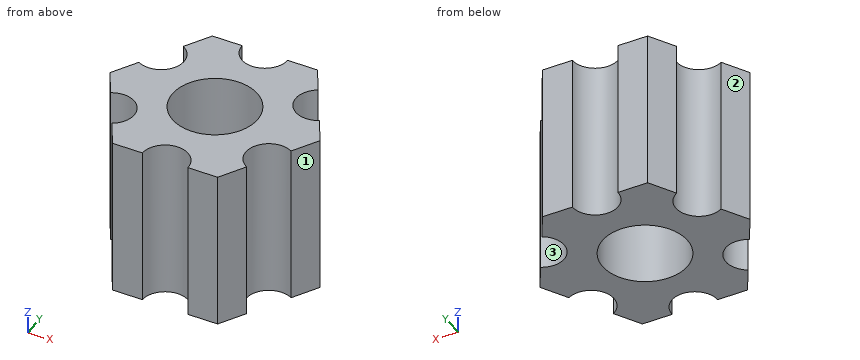
```python
from build123d import *

# Parameters (mm, degrees)
SKETCH1_R           = 2.9337
BOSS_EXTRUDE1_DEPTH = 15.875
CUT_EXTRUDE1_DEPTH  = 4.7625


with BuildPart() as part:
    # Sketch1 → Boss-Extrude1 (new body)
    with BuildSketch(Plane(origin=(0, 0, 0), x_dir=(-1, 0, 0), z_dir=(0, 0, -1))):
        with BuildLine():
            Line((-4.70551159, -4.549815043), (-3.666174521, -6.349999904))
            Line((-3.666174521, -6.349999904), (-1.587500385, -6.349999904))
            ThreePointArc((-1.587500385, -6.349999904), (-3.85e-07, -4.762499904), (1.587499615, -6.349999904))
            Line((1.587499615, -6.349999904), (3.666173825, -6.349999904))
            Line((3.666173825, -6.349999904), (4.705510942, -4.54981524))
            ThreePointArc((4.705510942, -4.54981524), (4.124445629, -2.381249907), (6.293010962, -1.800184594))
            Line((6.293010962, -1.800184594), (7.332348079, 7e-08))
            Line((7.332348079, 7e-08), (6.293011217, 1.800184685))
            ThreePointArc((6.293011217, 1.800184685), (4.124445939, 2.381250203), (4.705511457, 4.549815481))
            Line((4.705511457, 4.549815481), (3.666174521, 6.350000222))
            Line((3.666174521, 6.350000222), (1.587500385, 6.350000222))
            ThreePointArc((1.587500385, 6.350000222), (3.85e-07, 4.762500222), (-1.587499615, 6.350000222))
            Line((-1.587499615, 6.350000222), (-3.666173825, 6.350000222))
            Line((-3.666173825, 6.350000222), (-4.705511038, 4.549815614))
            ThreePointArc((-4.705511038, 4.549815614), (-4.124445841, 2.38125025), (-6.293011205, 1.800185053))
            Line((-6.293011205, 1.800185053), (-7.332348419, 4.44e-07))
            Line((-7.332348419, 4.44e-07), (-6.293011423, -1.80018429))
            ThreePointArc((-6.293011423, -1.80018429), (-4.12444613, -2.38124975), (-4.70551159, -4.549815043))
        make_face()
        Circle(SKETCH1_R, mode=Mode.SUBTRACT)
    extrude(amount=-BOSS_EXTRUDE1_DEPTH)

    # Sketch3 → Cut-Extrude1 (cut)
    with BuildSketch(Plane.XY.offset(15.875)):
        with BuildLine():
            Line((-4.705511457, 4.549815481), (-3.666174521, 6.350000222))
            Line((-3.666174521, 6.350000222), (-1.587500385, 6.350000222))
            ThreePointArc((-1.587500385, 6.350000222), (-3.85e-07, 4.762500222), (1.587499615, 6.350000222))
            Line((1.587499615, 6.350000222), (3.666173825, 6.350000222))
            Line((3.666173825, 6.350000222), (4.705511038, 4.549815614))
            ThreePointArc((4.705511038, 4.549815614), (4.124445841, 2.38125025), (6.293011205, 1.800185053))
            Line((6.293011205, 1.800185053), (7.332348419, 4.44e-07))
            Line((7.332348419, 4.44e-07), (6.293011423, -1.80018429))
            ThreePointArc((6.293011423, -1.80018429), (4.12444613, -2.38124975), (4.70551159, -4.549815043))
            Line((4.70551159, -4.549815043), (3.666174521, -6.349999904))
            Line((3.666174521, -6.349999904), (1.587500385, -6.349999904))
            ThreePointArc((1.587500385, -6.349999904), (3.85e-07, -4.762499904), (-1.587499615, -6.349999904))
            Line((-1.587499615, -6.349999904), (-3.666173825, -6.349999904))
            Line((-3.666173825, -6.349999904), (-4.705510942, -4.54981524))
            ThreePointArc((-4.705510942, -4.54981524), (-4.124445629, -2.381249907), (-6.293010962, -1.800184594))
            Line((-6.293010962, -1.800184594), (-7.332348079, 7e-08))
            Line((-7.332348079, 7e-08), (-6.293011217, 1.800184685))
            ThreePointArc((-6.293011217, 1.800184685), (-4.124445939, 2.381250203), (-4.705511457, 4.549815481))
        make_face()
    extrude(amount=-CUT_EXTRUDE1_DEPTH, mode=Mode.SUBTRACT)


solid = part.part
```
For this review, take the finished solid that the model builds, in its own axes (mm). Face numbers are marked on the shaded views. Give positions to 0.01 mm unless a question says otherwise; leave off trailing zeros. Write each loop counter-clockwise with the first axis right and the second up, starting at its lowest first coordinate (ties: lowest second). Pieces come first, ordered by that corner, then holes. Notation, with made-up numbers: M 37,23.5 L 78,23.5 A23 ccw 78,43.5 Z; hole C 66,78.25 d4. An arc over 180 degrees is marked long. Answer as a JSON object with one key per item and string values. Group by question number.
Item 1: Consider section C-C on y = 1. Write out the cut boundary in (x, z) (1 decimal), plus the area to 3 significant figures.
Item 2: Draft analysis for pull direction X (two halves, no side actions). For the marked faces 1, 2 and 3, state which applies: +X half, -X half, draft (parallel to the pull), parting line (faces both ways), or undercut.
Item 3: Consider section D-D on x = 4.25. Write out the cut boundary in (y, z), plus the area to 3 significant figures.
Item 4: For probe 1 along Y at (x, z) = (0, 4.5); probe 2 along Y at (x, z) = (-4.5, 2.25); probe 3 along Y at (x, z) = (-2.25, 4), list the stretches that pass through material, from the lowest coordinate up. Write a range as [from, to].
Item 5: Consider section B-B on x = 0. Write out the cut boundary in (y, z), plus the area to 3 significant figures.
Item 6: For pin 1 Ø1.5 at (x, z) = (0, 7) entering from +Y; pin 2 Ø3 at (y, z) = (-3.5, 7.5) entering from +X; pin 3 Ø1 at (x, y) = (-1, -1) entering from -Z; pin 4 Ø3 at (x, z) = (4.5, 4.5) entering from +Y, all flat-tipped, find the tip position at first contact; note any pin that passes through.
Check result:
{
 "1": {"outline": "M -6.8,0 L -2.8,0 L -2.8,11.1 L -6.8,11.1 Z; M 2.8,0 L 6.8,0 L 6.8,11.1 L 2.8,11.1 Z", "area": "88.8 mm^2"},
 "2": {"face 1": "+X half", "face 2": "-X half", "face 3": "undercut"},
 "3": {"outline": "M -5.34,0 L -4.15,0 L -4.15,11.11 L -5.34,11.11 Z; M -2.2,0 L 2.2,0 L 2.2,11.11 L -2.2,11.11 Z; M 4.15,0 L 5.34,0 L 5.34,11.11 L 4.15,11.11 Z", "area": "75.1 mm^2"},
 "4": {"probe 1": "y = [-4.76, -2.93], [2.93, 4.76]", "probe 2": "y = [-4.91, -4.41], [-1.94, 1.94], [4.41, 4.91]", "probe 3": "y = [-6.35, -1.88], [1.88, 6.35]"},
 "5": {"outline": "M -4.76,0 L -2.93,0 L -2.93,11.11 L -4.76,11.11 Z; M 2.93,0 L 4.76,0 L 4.76,11.11 L 2.93,11.11 Z", "area": "40.6 mm^2"},
 "6": {"pin 1": "stops at y = 4.95", "pin 2": "stops at x = 4.71", "pin 3": "passes through", "pin 4": "stops at y = 6.35"}
}
